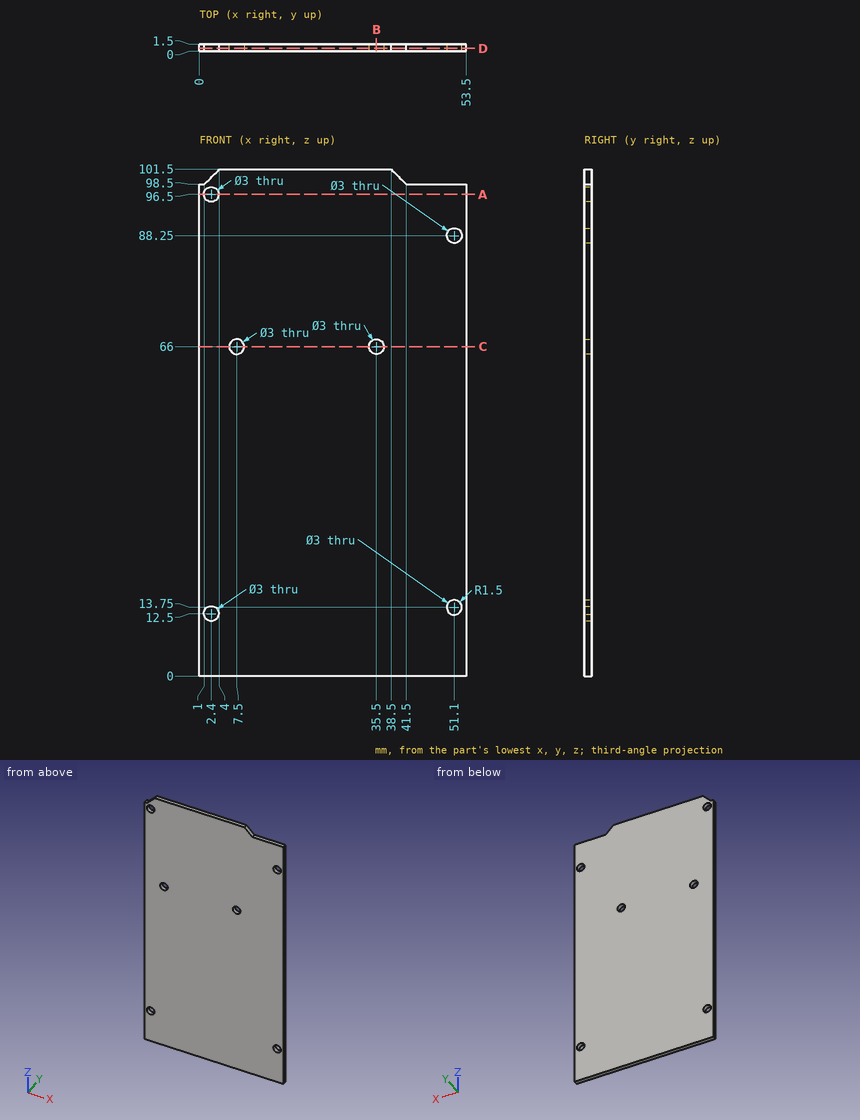
Source: three-view drawing plus pictorial views. Frame: mm from the lowest corner of the part. Round coordinates to 2 decimals unless told otherwise and drop trailing zeros. Order: outer loops, then holes, each group sorted by start corner. A loop starts at its lowest first (then second) coordinate and runs counter-clockwise, first axis right, second up. Notation, with made-up numbers: (47.25, -10.5) -> (82.25, -10.5) arc R29 cw to (82.25, 20.5) -> close; hole circle Ø7 at (7, 84.25). An arc over 180 degrees is marked (long way). Use one line per item in the form item = value.
(1) Section D-D on y = 0.6. Return loops of the section in (x, z), and give its area (3 significant figures).
Results list:
outline = (0, 0) -> (53.5, 0) -> (53.5, 98.5) -> (41.5, 98.5) -> (38.5, 101.5) -> (4, 101.5) -> (1, 98.5) -> (0, 98.5) -> close; hole circle Ø3 at (2.4, 12.5); hole circle Ø3 at (2.4, 96.5); hole circle Ø3 at (7.5, 66); hole circle Ø3 at (35.5, 66); hole circle Ø3 at (51.1, 13.75); hole circle Ø3 at (51.1, 88.25)
area = 5,340 mm^2
(2) First-contact query: pin 1 Ø2.5 at (x, z) = (35.5, 66) entering from -Y; pin 2 Ø0.5 at (x, y) = (0.5, 0.5) entering from +Z. Flat tips, straight axial feed; report the tip coordinate or a pass-through.
Results list:
pin_1 = through
pin_2 = 98.5
(3) Section A-A on z = 96.5. Return loops of the section in (x, y), and give its area (4 significant figures).
Results list:
outline = (0, 0) -> (0.9, 0) -> (0.9, 1.5) -> (0, 1.5) -> close; (3.9, 0) -> (53.5, 0) -> (53.5, 1.5) -> (3.9, 1.5) -> close
area = 75.75 mm^2
(4) Section B-B on x = 35.5. Return loops of the section in (y, z), and give its area (3 significant figures).
Results list:
outline = (0, 0) -> (1.5, 0) -> (1.5, 64.5) -> (0, 64.5) -> close; (0, 67.5) -> (1.5, 67.5) -> (1.5, 101.5) -> (0, 101.5) -> close
area = 148 mm^2
(5) Section C-C on z = 66. Return loops of the section in (x, y).
Results list:
outline = (0, 0) -> (6, 0) -> (6, 1.5) -> (0, 1.5) -> close; (9, 0) -> (34, 0) -> (34, 1.5) -> (9, 1.5) -> close; (37, 0) -> (53.5, 0) -> (53.5, 1.5) -> (37, 1.5) -> close
(6) Ray query, probe 1 along X at (y, z) = (0.6, 66); probe 2 along X at (y, z) = (0.9, 65.5); probe 3 along Z at (x, y) = (7.5, 1.25). Return the intervals inside material, ascending. Write a range as [from, to].
Results list:
probe_1 = [0, 6], [9, 34], [37, 53.5]
probe_2 = [0, 6.09], [8.91, 34.09], [36.91, 53.5]
probe_3 = [0, 64.5], [67.5, 101.5]
